The model under review builds one solid part; all positions refer to its coordinate system, in mm. A direction names the side the tool comes from. Coordinates: 2 decimals unless noted, no trailing zeros. Order: outer loops, then holes, each group sorted by start corner. A loop starts at its lowest first (then second) coordinate and runs counter-clockwise, first axis right, second up. Notation, with made-up numbers: M -19,27.25 L 14,27.25 A21 cw 14,63.25 Z; hole C -27.75,-39.5 d3. An arc over 180 degrees is marked long. Answer in a Markdown table with one row per item.
Autodesk Inventor part; units mm, degrees
ref_plane "YZ Plane" through (0, 0, 0) normal (1, 0, 0) x (0, 1, 0)
ref_plane "XZ Plane" through (0, 0, 0) normal (0, 1, 0) x (-1, 0, 0)
ref_plane "XY Plane" through (0, 0, 0) normal (0, 0, 1) x (1, 0, 0)
sketch "Sketch1" plane through (0, 0, 0) normal (1, 0, 0) x (0, 1, 0)
  line L0 (0, 0) -> (228.6, 0)
  line L1 (228.6, 0) -> (228.6, -35.56)
  line L2 (228.6, -35.56) -> (0, -35.56)
  line L3 (0, -35.56) -> (0, 0)
  line L4 (228.6, 0) -> (222.758, 0)
  line L5 (222.758, 0) -> (222.758, -35.56)
  line L6 (222.758, -35.56) -> (228.6, -35.56)
  line L7 (228.6, -35.56) -> (228.6, 0)
  circle A0 centre (224.79, -6.35) radius 1.5875
  circle A1 centre (224.79, -29.21) radius 1.5875
  line L8 (222.758, 0) -> (0, 0)
  line L9 (165.1, -5.08) -> (6.35, -5.08)
  line L10 (6.35, -5.08) -> (6.35, -30.48)
  line L11 (6.35, -30.48) -> (165.1, -30.48)
  line L12 (222.758, -33.02) -> (222.758, -2.54)
  line L13 (165.1, 0) -> (165.1, -35.56)
  line L14 (231.14, 2.54) -> (-2.54, 2.54)
  line L15 (-2.54, 2.54) -> (-2.54, -38.1)
  line L16 (-2.54, -38.1) -> (231.14, -38.1)
  line L17 (231.14, -38.1) -> (231.14, 2.54)
  point P0 (110.998, 0)
  point P1 (228.6, -17.78)
  dimension "d0" = 228.6
  dimension "d1" = 35.56
  dimension "d2" = 5.842
  dimension "d3" = 3.175
  dimension "d4" = 3.175
  dimension "d5" = 3.81
  dimension "d6" = 6.35
  dimension "d7" = 3.81
  dimension "d8" = 6.35
  dimension "d14" = 5.08
  dimension "d15" = 5.08
  dimension "d16" = 6.35
  dimension "d17" = 0
  dimension "d18" = 63.5
  dimension "d19" = 2.54
  dimension "d20" = 2.54
  dimension "d21" = 2.54
  dimension "d22" = 2.54
extrude "Extrusion1" add sketch "Sketch1" along normal blind 15.24 contours L0 L13 L9 L10 L11 L2 L3 | L0 L1 L2 L5
extrude "Extrusion2" add sketch "Sketch1" along normal blind 15.24 and the other way blind 2 contours L17 L16 L15 L14
sketch "Sketch2" plane through (15.24, 0, 0) normal (1, 0, 0) x (0, 0, -1)
  line L0 (5.08, 6.35) -> (5.08, 165.1)
  line L1 (30.48, 165.1) -> (30.48, 6.35)
  line L2 (30.48, 6.35) -> (5.08, 6.35)
  line L3 (5.08, 165.1) -> (30.48, 165.1)
  point P0 (0, 0)
extrude "Extrusion3" add sketch "Sketch2" against normal blind 6.35
sketch "Sketch3" plane through (0, 0, 0) normal (-1, 0, 0) x (0, 0, 1)
  circle A0 centre (-17.78, 45.72) radius 2.54
  circle A1 centre (-17.78, 45.72) radius 1.5875
  line L0 (0, 228.6) -> (0, 0)
  line L1 (0, 0) -> (-35.56, 0)
  circle A2 centre (-17.78, 102.616) radius 2.54
  circle A3 centre (-17.78, 102.616) radius 1.5875
  circle A4 centre (-17.78, 159.512) radius 2.54
  circle A5 centre (-17.78, 159.512) radius 1.5875
  circle A6 centre (-17.78, 3.81) radius 1.5875
  dimension "d29" = 5.08
  dimension "d30" = 3.175
  dimension "d31" = 17.78
  dimension "d32" = 45.72
  dimension "d33" = 5.08
  dimension "d34" = 3.175
  dimension "d35" = 102.616
  dimension "d36" = 5.08
  dimension "d37" = 3.175
  dimension "d38" = 159.512
  dimension "d39" = 17.78
  dimension "d40" = 17.78
  dimension "d42" = 3.175
extrude "Extrusion4" add sketch "Sketch3" against normal up to surface (8.89 mm away) contours A0 | A2 | A4
extrude "Extrusion5" cut sketch "Sketch3" against normal through all contours A1 | A3 | A5 | A6
sketch "Sketch4" plane through (-2, 231.14, 2.54) normal (0, 1, 0) x (1, 0, 0)
  line L0 (17.24, 40.64) -> (17.24, 0)
  line L1 (17.24, 0) -> (17.24, -12.7)
  line L2 (17.24, -12.7) -> (0, 0)
  line L3 (17.24, 40.64) -> (17.24, 53.34)
  line L4 (0, 40.64) -> (17.24, 40.64)
  line L5 (17.24, 53.34) -> (0, 40.64)
  line L6 (0, 0) -> (17.24, 0)
  point P0 (2, 2.54)
  dimension "d48" = 12.7
  dimension "d49" = 12.7
extrude "Extrusion6" add sketch "Sketch4" against normal up to surface (233.68 mm away)
properties part number "Fullenss sensor v3.1 holder"
(1) To check wall thickness, follow line 1 (Y direction, x = 11, z = -18); line 2 (Z direction, x = 7, y = 160.5); line 3 (Z direction, x = 11.5, y = 224.79). State the ranges of each line that lie inside material, in increasing order. Write a range as [from, to].
Report:
| item | result |
|---|---|
| line 1 | [-2.54, 2.24], [5.38, 44.15], [47.29, 101.04], [104.19, 157.94], [161.08, 165.1], [222.76, 231.14] |
| line 2 | [-44.73, -30.48], [-20.12, -19.02], [-16.54, -15.44], [-5.08, 9.17] |
| line 3 | [-48.04, -30.8], [-27.62, -7.94], [-4.76, 12.48] |
(2) The part is to be moulded in two halves that separate along Z. For faces 1 (the flat face through (-2, 113.8, 0.4)), 2 (the flat face through (0, 103, -16)), 3 (the flat face through (6.74, 115.94, -44.54)), 4 (the flat face through (6.74, 115.94, 8.98)), say which applies: +Z half, -Z half, draft (parallel to the pull), parting line (faces both ways), or undercut.
Report:
| item | result |
|---|---|
| face 1 | draft |
| face 2 | undercut |
| face 3 | -Z half |
| face 4 | +Z half |
(3) Take a section at A-A (z = -12). Write out the cut boundary in (x, y), then the cut area to 3 significant figures.
Report:
| item | result |
|---|---|
| outline | M -2,-2.54 L 15.24,-2.54 L 15.24,165.1 L 8.89,165.1 L 8.89,6.35 L 0,6.35 L 0,0 L -2,0 Z; M -2,228.6 L 0,228.6 L 0,222.76 L 15.24,222.76 L 15.24,231.14 L -2,231.14 Z |
| area | 1,280 mm^2 |
(4) Insertion check: P1, Ø6, axis at y = 108.5, z = -4, coming from the -X side; P2, Ø2, axis at y = 147.5, z = -19, coming from the -X side; P3, Ø1, axis at x = 2.5, y = 117, coming from the +Z side. Each pin has a flat end and moves straight along its axis. Give the tip position at first contact, or say it passes through.
Report:
| item | result |
|---|---|
| P1 | x = 0 |
| P2 | x = 8.89 |
| P3 | z = 6.22 |
(5) Take a section at B-B (x = 2.5). State how many separate pieces and enclosed holes the cut face has, then the cut area to 3 significant figures.
Report:
| item | result |
|---|---|
| separate pieces | 4 |
| enclosed holes | 7 |
| area | 4,980 mm^2 |
(6) Machinability: for faces 5 (the flat face through (6, -2.54, -17)), 6 (the flat face through (11, 165.1, -18)), 7 (the flat face through (0, 158, -19)), which of the approach directions +Z, -Z, +X, -X, +Y, -Y give a long, thin tool a straight path to every point of the face, cutting with its end or side? Answer none if there is none.
Report:
| item | result |
|---|---|
| face 5 | +Z, -Z, +X, -X, -Y |
| face 6 | +X, -X |
| face 7 | -X |
(7) Take a section at C-C (y = 199). Write out the cut boundary in (x, z), then the cut area to 3 significant figures.
Report:
| item | result |
|---|---|
| outline | M -2,-38.1 L 15.24,-50.8 L 15.24,-35.56 L -2,-35.56 Z; M -2,0 L 15.24,0 L 15.24,15.24 L -2,2.54 Z |
| area | 307 mm^2 |
(8) Take a section at D-D (y = 36.5). Write out the cut boundary in (x, z).
Report:
| item | result |
|---|---|
| outline | M -2,-38.1 L 15.24,-50.8 L 15.24,15.24 L -2,2.54 L -2,0 L 0,0 L 0,-5.08 L 8.89,-5.08 L 8.89,-30.48 L 0,-30.48 L 0,-35.56 L -2,-35.56 Z |
